from build123d import *

# Parameters (mm, degrees)
F1_W     = 75
F1_H     = 50
F2_DEPTH = 32.5
F3_W     = 70
F3_H     = 45
F3_W_2   = 0.1495928758
F3_H_2   = 0.0465683566
F4_DEPTH = 30
F5_R     = 10
F6_DEPTH = 76
F7_R     = 5


with BuildPart() as f2:
    # F1 (on Top) → F2 (new body)
    with BuildSketch(Plane.XY):
        Rectangle(F1_W, F1_H)
    extrude(amount=F2_DEPTH)

    # F3 (on face) → F4 (cut)
    with BuildSketch(Plane.XY.offset(32.5)):
        with Locations((0.0747964379, 0.0232841783)):
            Rectangle(F3_W, F3_H)
        Rectangle(F3_W_2, F3_H_2, mode=Mode.SUBTRACT)
    extrude(amount=-F4_DEPTH, mode=Mode.SUBTRACT)

    # F5 (on face) → F6 (cut)
    with BuildSketch(Plane.YZ.offset(37.5)):
        with Locations((0, 32.5)):
            Circle(F5_R)
        with BuildLine():
            ThreePointArc((-10, 32.5), (0, 22.5), (10, 32.5))
            Line((10, 32.5), (-10, 32.5))
        make_face()
    extrude(amount=-F6_DEPTH, mode=Mode.SUBTRACT)

    # F7
    f7_edges = [f2.edges().sort_by_distance(p)[0] for p in [
        (35.074796, -22.476716, 17.5),
        (0.074796, -22.476716, 2.5),
        (35.074796, 0.023284, 2.5),
        (-36.212602, -10, 32.5),
        (36.287398, -10, 32.5),
        (36.287398, 10, 32.5),
        (-36.212602, 10, 32.5),
        (35.074796, 22.523284, 17.5),
        (0.074796, 22.523284, 2.5),
        (-34.925204, 0.023284, 2.5),
        (-34.925204, -22.476716, 17.5),
        (-34.925204, 22.523284, 17.5),
    ]]
    fillet(f7_edges, radius=F7_R)


solid = f2.part
Model file for the job. Use its own axes, mm. A direction names the side the tool comes from. Coordinates: 2 decimals unless noted, no trailing zeros. Write each loop counter-clockwise with the first axis right and the second up, starting at its lowest first coordinate (ties: lowest second). Pieces come first, ordered by that corner, then holes. Notation, with made-up numbers: (55.5, 46.25) - (105.5, 46.25) arc R17 cw to (105.5, 53.25) - close; hole circle Ø3 at (43.5, 3.25). An arc over 180 degrees is marked (long way). Write each question's results on one line, items separated by ' | '. Start each with the question number.
1) Flat gauge pin, fed straight in: P1, Ø3, axis at x = -22.5, y = -1, coming from the +Z side. Where does the tip first touch, or does it go through?
2) 3-axis set-ups, long thin cutter, end or side, ignore diameter. For faces 4 (the face through (-34.925, 0, 17)), 5 (the face through (-1, 0, 0)), 6 (the face through (36.27, -11.291, 31.607)): which of +Z, -Z, +X, -X, +Y, -Y reach the whole face in a straight line?
3) Mould opens along X. For faces 1 (the face through (0, 23, 32.5)), 2 (the face through (0, 22.523, 20)), 3 (the face through (37.5, 0, 16)) say: pulls with the +X half, pulls with the -X half, needs draft (parallel to the pull), parting line crosses it, or undercut.
4) Cut at D-D (x = -21.5). Write the cut outline in (y, z).
5) Cut at A-A (z = 15.5). Write the cut outline in (x, y).
6) Cut at B-B (z = 30.5). Write the cut outline in (x, y).
7) Cut at C-C (y = 6). Write the cut outline in (x, z), then the cut area to 3 significant figures.
8) Probe line 1 along Y through (x, z) = (-4, 22); line 2 along X through (y, z) = (13.5, 25); line 3 along Z through (x, y) = (-12.5, -3.5). List the from-to ranges inside material, lowest first. Write a range as from..to.
Returned:
1) P1: z = 2.5
2) face 4: +Z | face 5: -Z, +X, -X, +Y, -Y | face 6: +Z, +X, -X
3) face 1: needs draft | face 2: undercut | face 3: pulls with the +X half
4) outline: (-25, 0) - (25, 0) - (25, 32.5) - (22.52, 32.5) - (22.52, 7.5) arc R5 cw to (17.52, 2.5) - (-17.48, 2.5) arc R5 cw to (-22.48, 7.5) - (-22.48, 32.5) - (-25, 32.5) - close
5) outline: (-37.5, -25) - (37.5, -25) - (37.5, 25) - (-37.5, 25) - close; (-0.07, -0.02) - (0.07, -0.02) - (0.07, 0.02) - (-0.07, 0.02) - close; hole (-34.93, -17.48) arc R5 ccw to (-29.93, -22.48) - (30.07, -22.48) arc R5 ccw to (35.07, -17.48) - (35.07, 17.52) arc R5 ccw to (30.07, 22.52) - (-29.93, 22.52) arc R5 ccw to (-34.93, 17.52) - close
6) outline: (-37.5, -25) - (37.5, -25) - (37.5, -10.14) - (35.07, -10.14) - (35.07, -17.48) arc R5 cw to (30.07, -22.48) - (-29.93, -22.48) arc R5 cw to (-34.93, -17.48) - (-34.93, -10.14) - (-37.5, -10.14) - close; (-37.5, 10.14) - (-34.93, 10.14) - (-34.93, 17.52) arc R5 cw to (-29.93, 22.52) - (30.07, 22.52) arc R5 cw to (35.07, 17.52) - (35.07, 10.14) - (37.5, 10.14) - (37.5, 25) - (-37.5, 25) - close
7) outline: (-37.5, 0) - (37.5, 0) - (37.5, 24.5) - (35.07, 24.5) - (35.07, 7.5) arc R5 cw to (30.07, 2.5) - (-29.93, 2.5) arc R5 cw to (-34.93, 7.5) - (-34.93, 24.5) - (-37.5, 24.5) - close | area: 308 mm^2
8) line 1: -25..-22.48, 22.52..25 | line 2: -37.5..-34.93, 35.07..37.5 | line 3: 0..2.5
